Geometry: final body of the model. Coordinates: model frame, mm. Face numbers are marked on the shaded views. Give positions to 0.01 mm unless a question says otherwise; leave off trailing zeros. Order: outer loops, then holes, each group sorted by start corner. A loop starts at its lowest first (then second) coordinate and runs counter-clockwise, first axis right, second up. Notation, with made-up numbers: (-30.5, -15) - (-1.5, -15) arc R18 cw to (-1.5, 3) - close; hole circle Ø4 at (-14, 85). An arc over 180 degrees is marked (long way). Put each result on its own line as item: value. Start each with the question number.
1. Section D-D on y = 7. Return the cut outline in (x, z) (3 decimals), plus the area to 3 significant figures.
2. Section C-C on y = -9.5. Return the cut outline in (x, z) (3 decimals).
3. Section B-B on z = 2.6. Return the cut outline in (x, y).
4. First-contact query: P1, Ø1, axis at x = -1.5, z = 2.5, coming from the -Y side; P2, Ø0.7, axis at y = -4.5, z = 1, coming from the +X side; P3, Ø0.8, axis at y = -5.5, z = 3, coming from the +X side. Flat tips, straight axial feed; report the tip coordinate or a pass-through.
5. Section A-A on x = 0. Return the cut outline in (y, z) (3 decimals).
6. Mould query, pull axis Y, two halves, no side actions, for the marked faces 1, 2 and 3. Classes: pulls with the +Y half, pulls with the -Y half, needs draft (parallel to the pull), parting line crosses it, or undercut.
7. Ray query, line 1 along Y through (x, z) = (0, 0.95); line 2 along X through (y, z) = (-6.25, 1.5); line 3 along X through (y, z) = (-7.5, 3.05). Return the intervals inside material, ascending. Write a range as from..to.
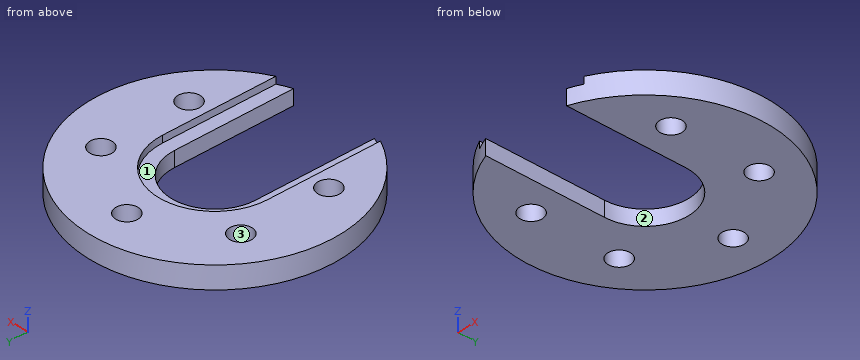
Autodesk Inventor part; units mm, degrees
ref_plane "YZ Plane" through (0, 0, 0) normal (1, 0, 0) x (0, 1, 0)
ref_plane "XZ Plane" through (0, 0, 0) normal (0, 1, 0) x (-1, 0, 0)
ref_plane "XY Plane" through (0, 0, 0) normal (0, 0, 1) x (1, 0, 0)
sketch "Sketch1" plane through (0, 0, 0) normal (0, 0, 1) x (1, 0, 0)
  arc A0 (6.25, 0) -> (-6.25, 0) centre (0, 0) ccw
  arc A1 (8.1, 0) -> (-8.1, 0) centre (0, 0) ccw
  arc A2 (8.1, -9.5205) -> (-8.1, -9.5205) centre (0, 0) ccw
  arc A3 (6.25, -16.8801) -> (-6.25, -16.8801) centre (0, 0) ccw
  line L0 (-6.25, 0) -> (-6.25, -16.8801)
  line L1 (6.25, 0) -> (6.25, -16.8801)
  line L2 (8.1, 0) -> (8.1, -16.0745)
  line L3 (-8.1, 0) -> (-8.1, -16.0745)
  circle A4 centre (0, 12.5) radius 1.6
  circle A5 centre (-10.8253, 6.25) radius 1.6
  circle A6 centre (-10.8253, -6.25) radius 1.6
  circle A7 centre (0, -12.5) radius 1.6
  circle A8 centre (10.8253, -6.25) radius 1.6
  circle A9 centre (10.8253, 6.25) radius 1.6
  dimension "d0" = 12.5
  dimension "d2" = 16.2
  dimension "d3" = 25
  dimension "d4" = 36
  dimension "d5" = 3.2
  dimension "d8" = 360
extrude "Extrusion1" add sketch "Sketch1" along normal blind 2.175 contours A0 L0 A3 L3 A1 L2 L1
extrude "Extrusion2" add sketch "Sketch1" along normal blind 3.175 contours L2 A2 A8 A9 A4 A5 A6 L3 A3 | L2 A1 L3 A2 A6 A5 A4 A9 A8 | A8 A2 | A2 A8 | A6 A2 | A2 A6 | A9 A2 | A2 A9 | A5 A2 | A2 A5 | A4 A2 | A2 A4
extrude "Extrusion3" cut sketch "Sketch1" along normal through all contours A8 A2 | A2 A8 | A6 A2 | A2 A6 | A9 A2 | A2 A9 | A5 A2 | A2 A5 | A4 A2 | A2 A4
equation "\"d12\" = THICKA"
equation "\"THICKA\" = 3.175"
equation "\"THICKB\" = 6.731"
equation "\"THICKC\" = 12.7"
equation "\"BALLDIA\" = 12"
equation "\"MAGDIA\" = 9.5"
equation "\"THICKPLY\" = 5"
properties part number "Effector_GrooveMount"
Resolved:
1. outline: (-16.583, 0) - (-12.239, 0) - (-12.239, 3.175) - (-16.583, 3.175) - close; (-9.412, 0) - (9.412, 0) - (9.412, 3.175) - (4.076, 3.175) - (4.076, 2.175) - (-4.076, 2.175) - (-4.076, 3.175) - (-9.412, 3.175) - close; (12.239, 0) - (16.583, 0) - (16.583, 3.175) - (12.239, 3.175) - close
1. area: 79.2 mm^2
2. outline: (-15.289, 0) - (-6.25, 0) - (-6.25, 2.175) - (-8.1, 2.175) - (-8.1, 3.175) - (-15.289, 3.175) - close; (6.25, 0) - (15.289, 0) - (15.289, 3.175) - (8.1, 3.175) - (8.1, 2.175) - (6.25, 2.175) - close
3. outline: (-8.1, -16.07) - (-8.1, 0) arc R8.1 cw to (8.1, 0) - (8.1, -16.07) arc R18 ccw (long way) to start; hole circle Ø3.2 at (-10.83, -6.25); hole circle Ø3.2 at (-10.83, 6.25); hole circle Ø3.2 at (0, 12.5); hole circle Ø3.2 at (10.83, -6.25); hole circle Ø3.2 at (10.83, 6.25)
4. P1: y = 5.96
4. P2: x = 17.52
4. P3: x = 17.26
5. outline: (6.25, 0) - (10.9, 0) - (10.9, 3.175) - (8.1, 3.175) - (8.1, 2.175) - (6.25, 2.175) - close; (14.1, 0) - (18, 0) - (18, 3.175) - (14.1, 3.175) - close
6. face 1: needs draft
6. face 2: pulls with the -Y half
6. face 3: undercut
7. line 1: 6.25..10.9, 14.1..18
7. line 2: -16.88..-12.43, -9.23..-6.25, 6.25..9.23, 12.43..16.88
7. line 3: -16.36..-11.82, -9.83..-8.1, 8.1..9.83, 11.82..16.36
